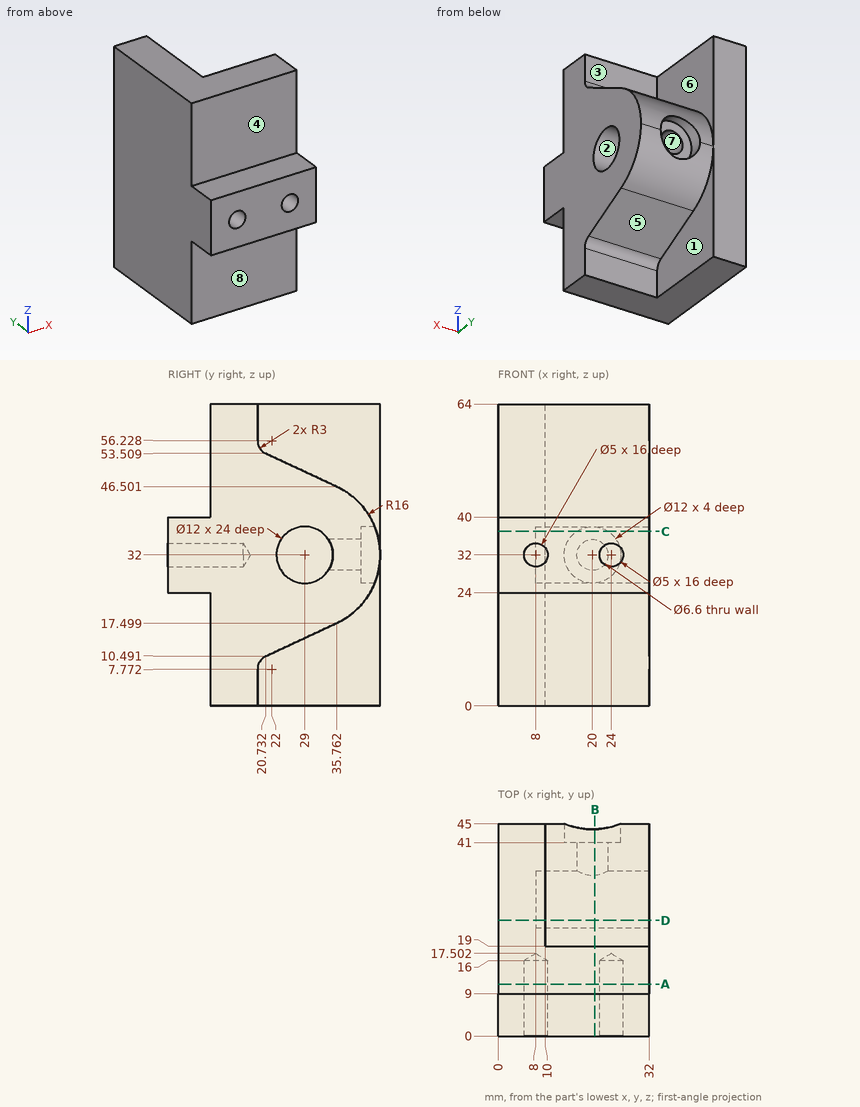
The figure shows three views and two pictorial views of one solid part (mm, origin at its lowest corner). Answer the questions. A direction names the side the tool comes from. Round coordinates to 2 decimals unless told otherwise and drop trailing zeros. Loops run counter-clockwise (first coordinate to the right, second up) from the corner with the lowest first, then second, coordinate; pieces in that order, holes last. Notation, with made-up numbers: M 66.5,66.25 L 107.5,66.25 A28 ccw 107.5,94.25 Z; hole C 70,56.5 d5. An arc over 180 degrees is marked long. Return JSON: item names as keys, results as strings.
Q1. The mould has two halves that part along Y. Classify the marked faces 1, 2 and 3: released by +Y, released by -Y, zero draft, split by the parting line, or undercut.
Results list:
{"face 1": "zero draft", "face 2": "undercut", "face 3": "released by +Y"}
Q2. Find the intervals of material crossed by line 1 along X through (y, z) = (8, 32); line 2 along Z through (x, y) = (8, 10.5); line 3 along X through (y, z) = (43, 43.5), in increasing order. Write a range as from..to.
Results list:
{"line 1": "x = 0..5.5, 10.5..21.5, 26.5..32", "line 2": "z = 0..29.5, 34.5..64", "line 3": "x = 0..10"}
Q3. Find section C-C, the plane z = 37. Determine the outline of the cut face in (x, y).
Results list:
{"outline": "M 0,0 L 32,0 L 32,25.68 L 8,25.68 L 8,32.32 L 32,32.32 L 32,44.2 L 23.32,44.2 L 23.32,41 L 16.68,41 L 16.68,44.2 L 10,44.2 L 10,45 L 0,45 Z"}
Q4. Find section D-D, the plane y = 24.5. Determine the outline of the cut face in (x, z).
Results list:
{"outline": "M 0,0 L 10,0 L 10,12.25 L 32,12.25 L 32,28.03 L 8,28.03 L 8,35.97 L 32,35.97 L 32,51.75 L 10,51.75 L 10,64 L 0,64 Z"}
Q5. Each of these flat-tipped pins is pushed along its axis until it touches: pin 1 Ø4 at (x, z) = (8, 32) entering from -Y; pin 2 Ø10 at (x, y) = (18.5, 3) entering from -Z; pin 3 Ø4 at (x, z) = (18, 62) entering from +Y. Where does it stop, or does it pass through?
Results list:
{"pin 1": "stops at y = 16.3", "pin 2": "stops at z = 24", "pin 3": "stops at y = 19"}
Q6. Which of the six approach directions +Z, -Z, +X, -X, +Y, -Y give full straight-line access (tool end or side, diameter ignored) to the marked faces 4, 5, 6, 7 and 8?
Results list:
{"face 4": "+Z, +X, -X, -Y", "face 5": "-Z, +X, +Y", "face 6": "+Z, +X, +Y", "face 7": "+Y", "face 8": "-Z, +X, -X, -Y"}
Q7. Find section B-B, the plane x = 20.5. Determine the outline of the cut face in (y, z), plus the area to 3 significant figures.
Results list:
{"outline": "M 0,24 L 9,24 L 9,0 L 19,0 L 19,7.77 A3 cw 20.73,10.49 L 35.76,17.5 A16 ccw 43.84,26.02 L 41,26.02 L 41,28.74 L 34.04,28.74 A6 cw long 34.04,35.26 L 41,35.26 L 41,37.98 L 43.84,37.98 A16 ccw 35.76,46.5 L 20.73,53.51 A3 cw 19,56.23 L 19,64 L 9,64 L 9,40 L 0,40 Z", "area": "1,400 mm2"}
Q8. Find section A-A, the plane y = 11. Determine the outline of the cut face in (x, z).
Results list:
{"outline": "M 0,0 L 32,0 L 32,64 L 0,64 Z; hole C 8,32 d5; hole C 24,32 d5"}
